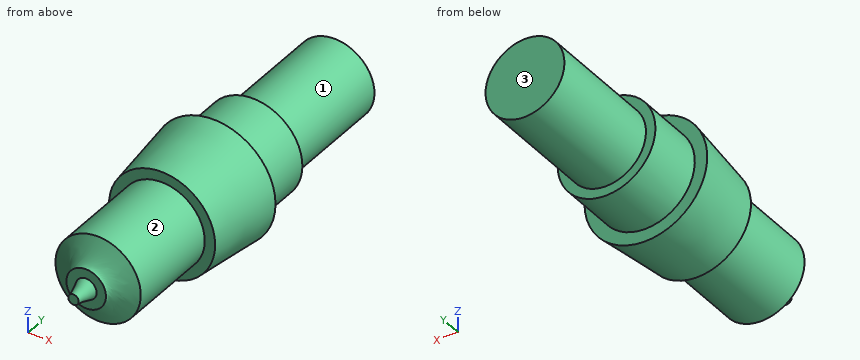
```python
from build123d import *

# Parameters (mm, degrees)
SKETCH1_R           = 18.95
BOSS_EXTRUDE1_DEPTH = 58
SKETCH2_R           = 23.5
BOSS_EXTRUDE2_DEPTH = 28
SKETCH3_R           = 29.5
SKETCH4_R           = 25.5
SKETCH6_R           = 20.5
BOSS_EXTRUDE3_DEPTH = 45.5


with BuildPart() as part:
    # Sketch1 → Boss-Extrude1 (new body)
    with BuildSketch(Plane(origin=(0, 0, 0), x_dir=(1, 0, 0), z_dir=(0, 1, 0))):
        with Locations(Location((0, 0, 0), (0, 0, 90))):
            Circle(SKETCH1_R)
    extrude(amount=BOSS_EXTRUDE1_DEPTH)

    # Sketch2 → Boss-Extrude2 (add)
    with BuildSketch(Plane.XZ):
        with Locations(Location((0, 0, 0), (0, 0, 270))):
            Circle(SKETCH2_R)
    extrude(amount=BOSS_EXTRUDE2_DEPTH)

    # Sketch3 → Loft1 section 0
    with BuildSketch(Plane.XZ.offset(28)):
        Circle(SKETCH3_R)
    # Sketch4 → Loft1 section 1
    with BuildSketch(Plane(origin=(0, -65, 0), x_dir=(-1, 0, 0), z_dir=(0, -1, 0))):
        Circle(SKETCH4_R)
    loft()

    # Sketch6 → Boss-Extrude3 (add)
    with BuildSketch(Plane.XZ.offset(65)):
        with Locations(Location((0, 0, 0), (0, 0, 270))):
            Circle(SKETCH6_R)
    extrude(amount=BOSS_EXTRUDE3_DEPTH)

    # Loft2: read off the stored shape, not the designer's step
    # Loft2: loft between two sections, ruled curve by curve
    loft2_from = [
        Edge.make_bspline([(19.32271694, -110.5, -6.847087705), (33.01689235, -110.5, 31.798346176), (-5.628541531, -110.5, 45.492521586), (-19.32271694, -110.5, 6.847087705), (-33.01689235, -110.5, -31.798346176), (5.628541531, -110.5, -45.492521586), (19.32271694, -110.5, -6.847087705)], [0, 0, 0, 0, 0.5, 0.5, 0.5, 1, 1, 1, 1], 3, [1, 0.333333333, 0.333333333, 1, 0.333333333, 0.333333333, 1]),
    ]
    loft2_to = [
        Edge.make_bspline([(6.801396589, -119, 6.63257148), (-6.463746372, -119, 20.235364658), (-20.06653955, -119, 6.970221697), (-6.801396589, -119, -6.63257148), (6.463746372, -119, -20.235364658), (20.06653955, -119, -6.970221697), (6.801396589, -119, 6.63257148)], [0, 0, 0, 0, 0.5, 0.5, 0.5, 1, 1, 1, 1], 3, [1, 0.333333333, 0.333333333, 1, 0.333333333, 0.333333333, 1]),
    ]
    loft2 = Solid(Shell([*[Face.make_surface_from_curves(loft2_from[k], loft2_to[k]) for k in range(1)], Face(Wire(loft2_from)), Face(Wire(loft2_to))]))
    add(loft2)

    # Loft5: read off the stored shape, not the designer's step
    # Loft5: loft between two sections, ruled curve by curve
    loft5_from = [
        Edge.make_bspline([(-4.99352595, -119, -0.254359166), (-4.484807619, -119, -10.241411066), (5.502244282, -119, -9.732692735), (4.99352595, -119, 0.254359166), (4.484807619, -119, 10.241411066), (-5.502244282, -119, 9.732692735), (-4.99352595, -119, -0.254359166)], [0, 0, 0, 0, 0.5, 0.5, 0.5, 1, 1, 1, 1], 3, [1, 0.333333333, 0.333333333, 1, 0.333333333, 0.333333333, 1]),
    ]
    loft5_to = [
        Edge.make_bspline([(-1.785448857, -128, 1.749906392), (-5.28526164, -128, -1.820991321), (-1.714363927, -128, -5.320804105), (1.785448857, -128, -1.749906392), (5.28526164, -128, 1.820991321), (1.714363927, -128, 5.320804105), (-1.785448857, -128, 1.749906392)], [0, 0, 0, 0, 0.5, 0.5, 0.5, 1, 1, 1, 1], 3, [1, 0.333333333, 0.333333333, 1, 0.333333333, 0.333333333, 1]),
    ]
    loft5 = Solid(Shell([*[Face.make_surface_from_curves(loft5_from[k], loft5_to[k]) for k in range(1)], Face(Wire(loft5_from)), Face(Wire(loft5_to))]))
    add(loft5)


solid = part.part
```
The model under review builds one solid part; all positions refer to its coordinate system, in mm. Face numbers are marked on the shaded views. A direction names the side the tool comes from. Coordinates: 2 decimals unless noted, no trailing zeros. Loops run counter-clockwise (first coordinate to the right, second up) from the corner with the lowest first, then second, coordinate; pieces in that order, holes last. Notation, with made-up numbers: (-19, -28) -> (9, -28) arc R24 cw to (9, 2) -> close; hole circle Ø4 at (-14.5, 28.25). An arc over 180 degrees is marked (long way). Answer as CSV lines item,"result".
Item 1: Insertion check: pin 1 (1.5 mm diameter, centred on x = -0.5, y = -102.5, fed in from -Z); pin 2 (8 mm diameter, centred on x = 17, z = -21.5, fed in from -Y); pin 3 (2 mm diameter, centred on x = 20.5, y = -41, fed in from +Z). Each pin has a flat end and moves straight along its axis. Give the tip position at first contact, or say it passes through.
Results below:
pin 1,"stops at z = -20.5"
pin 2,"stops at y = -65"
pin 3,"stops at z = 20.24"
Item 2: Take a section at A-A, the plane y = -91. State the section outline as (x, z) points.
Results below:
outline,"circle Ø41 at (0, 0)"
Item 3: For L1, parallel to Y at x = 8.5, z = -1; L2, parallel to Y at x = 23, z = 9; L3, parallel to X at y = -56.5, z = -7, list the stretches that pass through material, from the lowest coordinate up.
Results below:
L1,"y = -119 to 58"
L2,"y = -65 to -28"
L3,"x = -25.47 to 25.47"
Item 4: Machinability: for the marked faces 1, 2 and 3, which of the approach directions +Z, -Z, +X, -X, +Y, -Y give a long, thin tool a straight path to every point of the face, cutting with its end or side? Answer none if there is none.
Results below:
face 1,"+Y"
face 2,"-Y"
face 3,"+Z, -Z, +X, -X, +Y"
Item 5: Take a section at B-B, the plane y = -32. State the section outline as (x, z) points, and give its area (3 significant figures).
Results below:
outline,"circle Ø58.14 at (0, 0)"
area,"2,650 mm2"
